Input: part model. Units: mm. Frame: model coordinates. A direction names the side the tool comes from. Coordinates: 2 decimals unless noted, no trailing zeros. Loops run counter-clockwise (first coordinate to the right, second up) from the corner with the lowest first, then second, coordinate; pieces in that order, holes last. Notation, with made-up numbers: (86, -14) -> (131, -14) arc R13 ccw to (131, 7) -> close; hole circle Ø5 at (83.5, -26.5). An arc over 180 degrees is marked (long way). Answer as a JSON object with one key per item and string values.
from build123d import *

# Parameters (mm, degrees)
F0_W     = 275.00072
F0_H     = 101.6
F1_DEPTH = 177.8
F2_R     = 5
F3_DEPTH = 25
F4_W     = 168.275
F4_H     = 92.075
F5_DEPTH = 275.00172
F6_R     = 5
F7_DEPTH = 25.4


with BuildPart() as f1:
    # F0 (on Front) → F1 (new body)
    with BuildSketch(Plane.XZ):
        with Locations((-10.94948, -102.961591)):
            Rectangle(F0_W, F0_H)
    extrude(amount=F1_DEPTH)

    # F2 (on face) → F3 (cut)
    with BuildSketch(Plane.XZ.offset(177.8)):
        with Locations((-130.14984, -60.073791)):
            Circle(F2_R)
        with Locations((-130.14984, -132.073791)):
            Circle(F2_R)
        with Locations((108.25088, -132.073791)):
            Circle(F2_R)
        with Locations((108.25088, -60.073791)):
            Circle(F2_R)
    extrude(amount=-F3_DEPTH, mode=Mode.SUBTRACT)

    # F4 (on face) → F5 (cut, through all)
    with BuildSketch(Plane(origin=(-148.44984, 0, 0), x_dir=(0, -1, 0), z_dir=(-1, 0, 0))):
        with Locations((84.1375, -98.199091)):
            Rectangle(F4_W, F4_H)
    extrude(amount=-F5_DEPTH, mode=Mode.SUBTRACT)

    # F6 (on face) → F7 (cut)
    with BuildSketch(Plane(origin=(0, 0, -153.761591), x_dir=(1, 0, 0), z_dir=(0, 0, -1))):
        with Locations((8.10052, 34.4795)):
            Circle(F6_R)
        with Locations((-29.99948, 34.4795)):
            Circle(F6_R)
    extrude(amount=-F7_DEPTH, mode=Mode.SUBTRACT)


solid = f1.part
1. Section query C-C (y = -83). Return loops of the section in (x, z).
Reply:
{"outline": "(-148.45, -153.76) -> (126.55, -153.76) -> (126.55, -144.24) -> (-148.45, -144.24) -> close"}
2. Line query: line 1 along X through (y, z) = (-168.5, -60); line 2 along Y through (x, z) = (99.5, -66) (3 decimals); line 3 along Z through (x, y) = (-127.5, -128). Output: solid intervals per line, ascending.
Reply:
{"line 1": "x = -148.45 to -135.15, -125.15 to 103.25, 113.25 to 126.55", "line 2": "y = -177.8 to -168.275", "line 3": "z = -153.76 to -144.24"}
3. Access query for faces 1 (the face through (-13, -168.275, -99)), 2 (the face through (-13, -177.8, -102)). Directions: +Z, -Z, +X, -X, +Y, -Y. A direction counts if a zero-diameter tool reaches every point of the face in a straight line with its end or side. Return the directions, or none.
Reply:
{"face 1": "+Z, +X, -X, +Y", "face 2": "+Z, -Z, +X, -X, -Y"}
4. Section query B-B (z = -70.5). Return loops of the section in (x, y) (3 decimals).
Reply:
{"outline": "(-148.45, -177.8) -> (126.551, -177.8) -> (126.551, -168.275) -> (-148.45, -168.275) -> close"}
5. Pin query (flat end, axial travel): P1, Ø6, axis at x = 46, y = -93.5, coming from the +Z side; P2, Ø9, axis at x = 108.25, z = -60.07, coming from the +Y side; P3, Ø11.5, axis at x = -130.15, z = -132.07, coming from the +Y side (3 decimals). Return the tip coordinate at first contact, or that it passes through.
Reply:
{"P1": "stops at z = -144.24", "P2": "passes through", "P3": "stops at y = -168.275"}
6. Section query A-A (x = 97). Return loops of the section in (y, z) (3 decimals), plus the area to 3 significant figures.
Reply:
{"outline": "(-177.8, -153.762) -> (0, -153.762) -> (0, -144.237) -> (-168.275, -144.237) -> (-168.275, -52.162) -> (-177.8, -52.162) -> close", "area": "2,570 mm2"}
7. Mould query, pull axis Z, two halves, no side actions, for faces 3 (the face through (4.13, -31.44, -149.07)), 4 (the face through (-13, -88, -153.762)), 5 (the face through (110.56, -173.1, -136.51)). Classes: pulls with the +Z half, pulls with the -Z half, needs draft (parallel to the pull), parting line crosses it, or undercut.
Reply:
{"face 3": "needs draft", "face 4": "pulls with the -Z half", "face 5": "undercut"}
